```python
from build123d import *

# Parameters (mm, degrees)
ESTRUSIONE_ESTRUSIONE1_DEPTH = 120
TAGLIO_ESTRUSIONE2_REACH     = 166.924
SCHIZZO6_R                   = 6
TAGLIO_ESTRUSIONE3_REACH     = 166.924
SCHIZZO7_R                   = 9.5
FORO_PER_VITE_M4_2_D         = 4.5
SCHIZZO12_R                  = 3
TAGLIO_ESTRUSIONE4_DEPTH     = 10
SCHIZZO14_R                  = 2.6
TAGLIO_ESTRUSIONE5_DEPTH     = 10
SMUSSO2_SIZE                 = 1


with BuildPart() as part:
    # Schizzo1 → Estrusione-Estrusione1 (new body)
    with BuildSketch(Plane.XY):
        Polygon((0, 0), (-80, 0), (-80, -8), (-8, -8), (-8, -80), (0, -80), align=None)
    extrude(amount=ESTRUSIONE_ESTRUSIONE1_DEPTH)

    # Schizzo6 → Taglio-Estrusione2 (cut, up to next)
    with BuildSketch(Plane(origin=(0, 0, 0), x_dir=(1, 0, 0), z_dir=(0, 1, 0)), mode=Mode.PRIVATE) as taglio_estrusione2_sk1:
        with Locations(Location((-21, -21, 0), (0, 0, 180))):
            Circle(SCHIZZO6_R)
    taglio_estrusione2_tool1 = extrude(taglio_estrusione2_sk1.sketch, amount=-TAGLIO_ESTRUSIONE2_REACH, mode=Mode.PRIVATE) & part.part
    # Schizzo6 → Taglio-Estrusione2 (cut, up to next)
    with BuildSketch(Plane(origin=(0, 0, 0), x_dir=(1, 0, 0), z_dir=(0, 1, 0)), mode=Mode.PRIVATE) as taglio_estrusione2_sk2:
        with Locations(Location((-21, -99, 0), (0, 0, 180))):
            Circle(SCHIZZO6_R)
    taglio_estrusione2_tool2 = extrude(taglio_estrusione2_sk2.sketch, amount=-TAGLIO_ESTRUSIONE2_REACH, mode=Mode.PRIVATE) & part.part
    add(taglio_estrusione2_tool1.solids().sort_by_distance((-21, 0, 21))[0], mode=Mode.SUBTRACT)
    add(taglio_estrusione2_tool2.solids().sort_by_distance((-21, 0, 99))[0], mode=Mode.SUBTRACT)

    # Schizzo7 → Taglio-Estrusione3 (cut, up to next)
    with BuildSketch(Plane(origin=(0, 0, 0), x_dir=(1, 0, 0), z_dir=(0, 1, 0)), mode=Mode.PRIVATE) as taglio_estrusione3_sk1:
        with Locations(Location((-29, -60, 0), (0, 0, 180))):
            Circle(SCHIZZO7_R)
    taglio_estrusione3_tool1 = extrude(taglio_estrusione3_sk1.sketch, amount=-TAGLIO_ESTRUSIONE3_REACH, mode=Mode.PRIVATE) & part.part
    add(taglio_estrusione3_tool1.solids().sort_by_distance((-29, 0, 60))[0], mode=Mode.SUBTRACT)

    # Foro per Vite M4-2 (through all)
    with Locations(Plane(origin=(0, 0, 0), x_dir=(1, 0, 0), z_dir=(0, 1, 0))):
        with Locations((-29, -47), (-42, -60), (-29, -73), (-16, -60), (-29, -60)):
            Hole(FORO_PER_VITE_M4_2_D / 2)

    # Schizzo12 → Taglio-Estrusione4 (cut)
    with BuildSketch(Plane(origin=(0, 0, 0), x_dir=(0, 0, -1), z_dir=(1, 0, 0))):
        with Locations((-35, -73)):
            Circle(SCHIZZO12_R)
        with Locations(Location((-7, -73, 0), (0, 0, 90))):
            Circle(SCHIZZO12_R)
        with Locations((-113, -73)):
            Circle(SCHIZZO12_R)
        with Locations(Location((-85, -73, 0), (0, 0, 90))):
            Circle(SCHIZZO12_R)
        with Locations((-85, -52)):
            Circle(SCHIZZO12_R)
        with Locations(Location((-113, -52, 0), (0, 0, 90))):
            Circle(SCHIZZO12_R)
        with Locations(Location((-35, -52, 0), (0, 0, 90))):
            Circle(SCHIZZO12_R)
        with Locations((-7, -52)):
            Circle(SCHIZZO12_R)
        with Locations((-85, -16)):
            Circle(SCHIZZO12_R)
        with Locations(Location((-113, -16, 0), (0, 0, 90))):
            Circle(SCHIZZO12_R)
        with Locations((-35, -37)):
            Circle(SCHIZZO12_R)
        with Locations(Location((-7, -37, 0), (0, 0, 90))):
            Circle(SCHIZZO12_R)
        with Locations(Location((-35, -16, 0), (0, 0, 90))):
            Circle(SCHIZZO12_R)
        with Locations((-7, -16)):
            Circle(SCHIZZO12_R)
        with Locations(Location((-85, -37, 0), (0, 0, 90))):
            Circle(SCHIZZO12_R)
        with Locations((-113, -37)):
            Circle(SCHIZZO12_R)
    extrude(amount=-TAGLIO_ESTRUSIONE4_DEPTH, mode=Mode.SUBTRACT)

    # Schizzo14 → Taglio-Estrusione5 (cut)
    with BuildSketch(Plane(origin=(0, 0, 0), x_dir=(1, 0, 0), z_dir=(0, 1, 0))):
        with Locations(Location((-70, -18, 0), (0, 0, 180))):
            Circle(SCHIZZO14_R)
        with Locations(Location((-70, -60, 0), (0, 0, 180))):
            Circle(SCHIZZO14_R)
        with Locations(Location((-70, -102, 0), (0, 0, 180))):
            Circle(SCHIZZO14_R)
        with Locations(Location((-55, -35, 0), (0, 0, 180))):
            Circle(SCHIZZO14_R)
        with Locations(Location((-55, -85, 0), (0, 0, 180))):
            Circle(SCHIZZO14_R)
    extrude(amount=-TAGLIO_ESTRUSIONE5_DEPTH, mode=Mode.SUBTRACT)

    # Smusso2
    smusso2_edges = [part.edges().sort_by_distance(p)[0] for p in [
        (-19.5, 0, 60),
    ]]
    chamfer(smusso2_edges, length=SMUSSO2_SIZE)


solid = part.part
```
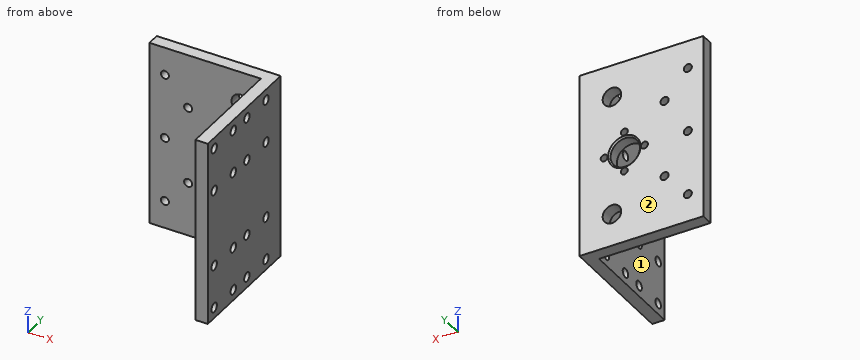
Geometry check sheet. Reference: the model listing, model coordinates, mm. Face numbers are marked on the shaded views. A direction names the side the tool comes from. Coordinates: 2 decimals unless noted, no trailing zeros. Write each loop counter-clockwise with the first axis right and the second up, starting at its lowest first coordinate (ties: lowest second). Pieces come first, ordered by that corner, then holes. Notation, with made-up numbers: M 5.5,75 L 45.5,75 A32 ccw 45.5,105 Z; hole C 52.25,-21.5 d4. An arc over 180 degrees is marked long. Answer as a JSON object with one key per item and string values.
1. Section check A-A, the plane z = 35. Enter the section's corners in (x, y).
Answers below:
{"outline": "M -80,-8 L -57.6,-8 L -57.6,0 L -80,0 Z; M -52.4,-8 L -8,-8 L -8,-13 L 0,-13 L 0,0 L -52.4,0 Z; M -8,-80 L 0,-80 L 0,-76 L -8,-76 Z; M -8,-70 L 0,-70 L 0,-55 L -8,-55 Z; M -8,-49 L 0,-49 L 0,-40 L -8,-40 Z; M -8,-34 L 0,-34 L 0,-19 L -8,-19 Z"}
2. Go/stop test with flat-tipped pins: pin 1 Ø9.5 at (y, z) = (-52, 7) entering from -X; pin 2 Ø6 at (y, z) = (-26, 62.5) entering from +X; pin 3 Ø6 at (x, z) = (-42, 60) entering from -Y; pin 4 Ø5 at (y, z) = (-73, 85) entering from +X. Record where each tip stops, or that it passes through.
Answers below:
{"pin 1": "stops at x = -8", "pin 2": "stops at x = 0", "pin 3": "stops at y = -8", "pin 4": "passes through"}
3. Scan lines: L1, parallel to X at y = -1, z = 47; L2, parallel to Y at x = -31, z = 40. Record each from-to range of solid material in increasing order.
Answers below:
{"L1": "x = -80 to -31.25, -26.75 to 0", "L2": "y = -8 to 0"}
4. Section check D-D, the plane z = 7. Enter the section's corners in (x, y), plus the area to 3 significant figures.
Answers below:
{"outline": "M -80,-8 L -8,-8 L -8,-13 L 0,-13 L 0,0 L -80,0 Z; M -8,-80 L 0,-80 L 0,-76 L -8,-76 Z; M -8,-70 L 0,-70 L 0,-55 L -8,-55 Z; M -8,-49 L 0,-49 L 0,-40 L -8,-40 Z; M -8,-34 L 0,-34 L 0,-19 L -8,-19 Z", "area": "1,020 mm²"}
5. Section check C-C, the plane y = -37. Enter the section's corners in (x, z), plus the area to 3 significant figures.
Answers below:
{"outline": "M -8,0 L 0,0 L 0,4 L -8,4 Z; M -8,10 L 0,10 L 0,32 L -8,32 Z; M -8,38 L 0,38 L 0,82 L -8,82 Z; M -8,88 L 0,88 L 0,110 L -8,110 Z; M -8,116 L 0,116 L 0,120 L -8,120 Z", "area": "768 mm²"}
6. Tool access check on the marked faces 1 and 2. Record the directions out of +Z, -Z, +X, -X, +Y, -Y that give a thin tool (end or side, any length) a straight path to the whole face; none if there is none.
Answers below:
{"face 1": "+Z, -Z, -X, -Y", "face 2": "+Z, -Z, +X, -X, +Y"}
7. Section check B-B, the plane x = -42. Enter the section's corners in (y, z), plus the area to 3 significant figures.
Answers below:
{"outline": "M -8,0 L 0,0 L 0,57.75 L -8,57.75 Z; M -8,62.25 L 0,62.25 L 0,120 L -8,120 Z", "area": "924 mm²"}
